Source: three-view drawing plus pictorial views. Frame: mm from the lowest corner of the part. A direction names the side the tool comes from. Round coordinates to 2 decimals unless told otherwise and drop trailing zeros. Loops run counter-clockwise (first coordinate to the right, second up) from the corner with the lowest first, then second, coordinate; pieces in that order, holes last. Notation, with made-up numbers: (-34, 32.25) -> (25, 32.25) arc R31 ccw to (25, 70.25) -> close; hole circle Ø1 at (79, 29). An arc over 180 degrees is marked (long way). Answer in a Markdown table with one row per item.
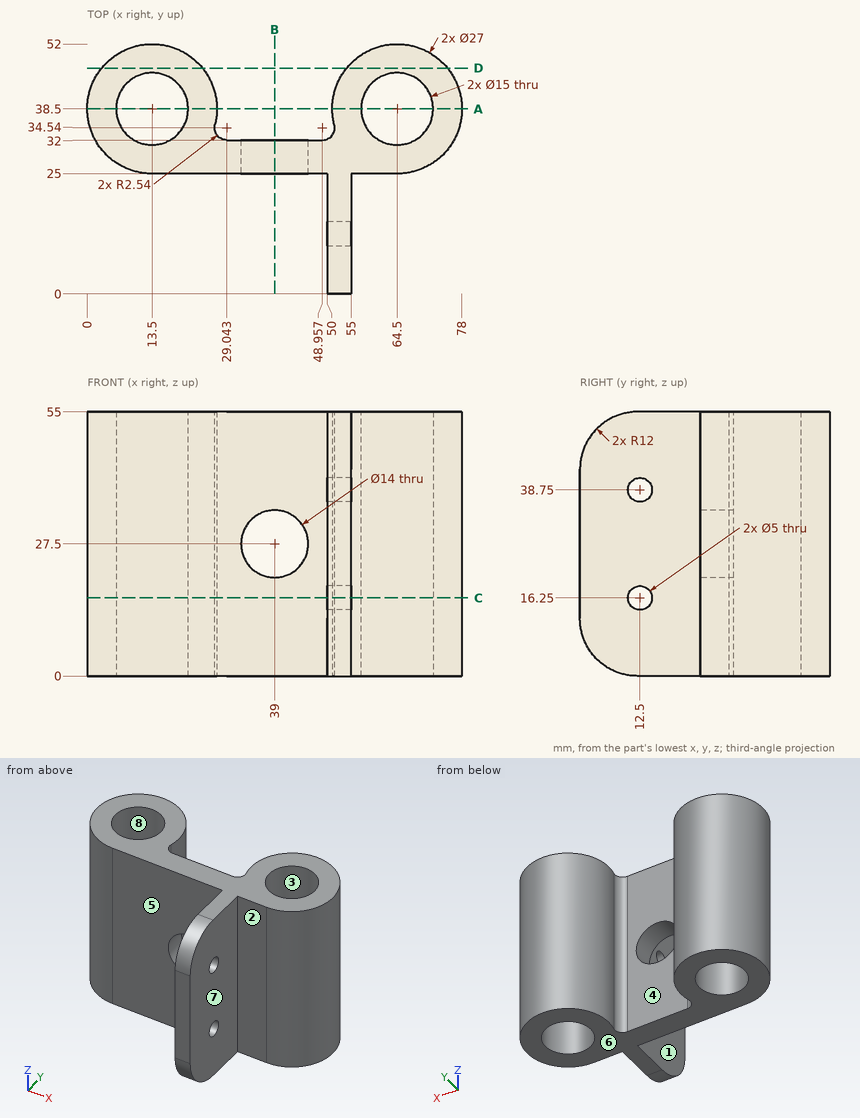
Item 1: Line query: probe 1 along Z at (x, y) = (53.1, 12.5); probe 2 along X at (y, z) = (38, 36); probe 3 along X at (y, z) = (4, 41). Output: solid intervals per line, ascending. Write a range as [from, to].
Answer:
| item | result |
|---|---|
| probe 1 | z = [0, 13.75], [18.75, 36.25], [41.25, 55] |
| probe 2 | x = [0.01, 6.02], [20.98, 26.99], [51.01, 57.02], [71.98, 77.99] |
| probe 3 | x = [50, 55] |
Item 2: Pin query (flat end, axial travel): pin 1 Ø7.5 at (y, z) = (8.5, 38) entering from -X; pin 2 Ø2 at (x, z) = (28, 12) entering from -Y; pin 3 Ø4 at (y, z) = (33.5, 32.5) entering from +X. Return the tip coordinate at first contact, or that it passes through.
Answer:
| item | result |
|---|---|
| pin 1 | stops at x = 50 |
| pin 2 | stops at y = 25 |
| pin 3 | stops at x = 77.66 |
Item 3: Cut plane C-C (z = 16.25). Output: boundary loops of the cut face in (x, y).
Answer:
| item | result |
|---|---|
| outline | (13.5, 25) -> (50, 25) -> (50, 15) -> (55, 15) -> (55, 25) -> (64.5, 25) arc R13.5 ccw (long way) to (51.42, 35.17) arc R2.54 cw to (48.96, 32) -> (29.04, 32) arc R2.54 cw to (26.58, 35.17) arc R13.5 ccw (long way) to start; (50, 0) -> (55, 0) -> (55, 10) -> (50, 10) -> close; hole circle Ø15 at (13.5, 38.5); hole circle Ø15 at (64.5, 38.5) |
Item 4: Reachability of the marked faces 4, 5, 6, 7 and 8 from +Z, -Z, +X, -X, +Y, -Y: full face, straight path, thin tool, end or side. Return the list, or none.
Answer:
| item | result |
|---|---|
| face 4 | +Z, -Z, +Y |
| face 5 | +Z, -Z, -X, -Y |
| face 6 | -Z, +X, -X, +Y, -Y |
| face 7 | +Z, -Z, +X, -Y |
| face 8 | +Z, -Z |
Item 5: Cut plane B-B (x = 39). Output: boundary loops of the cut face in (y, z).
Answer:
| item | result |
|---|---|
| outline | (25, 0) -> (32, 0) -> (32, 20.5) -> (25, 20.5) -> close; (25, 34.5) -> (32, 34.5) -> (32, 55) -> (25, 55) -> close |
Item 6: Cut plane D-D (y = 47). Output: boundary loops of the cut face in (x, z).
Answer:
| item | result |
|---|---|
| outline | (3.01, 0) -> (23.99, 0) -> (23.99, 55) -> (3.01, 55) -> close; (54.01, 0) -> (74.99, 0) -> (74.99, 55) -> (54.01, 55) -> close |
Item 7: Draft query along Y for the marked faces 1, 2 and 3. Return one class per face: pulls with the +Y half, pulls with the -Y half, needs draft (parallel to the pull), parting line crosses it, or undercut.
Answer:
| item | result |
|---|---|
| face 1 | needs draft |
| face 2 | pulls with the -Y half |
| face 3 | undercut |
Item 8: Cut plane A-A (y = 38.5). Output: boundary loops of the cut face in (x, z), then the cut area to 3 significant figures.
Answer:
| item | result |
|---|---|
| outline | (0, 0) -> (6, 0) -> (6, 55) -> (0, 55) -> close; (21, 0) -> (27, 0) -> (27, 55) -> (21, 55) -> close; (51, 0) -> (57, 0) -> (57, 55) -> (51, 55) -> close; (72, 0) -> (78, 0) -> (78, 55) -> (72, 55) -> close |
| area | 1,320 mm² |
